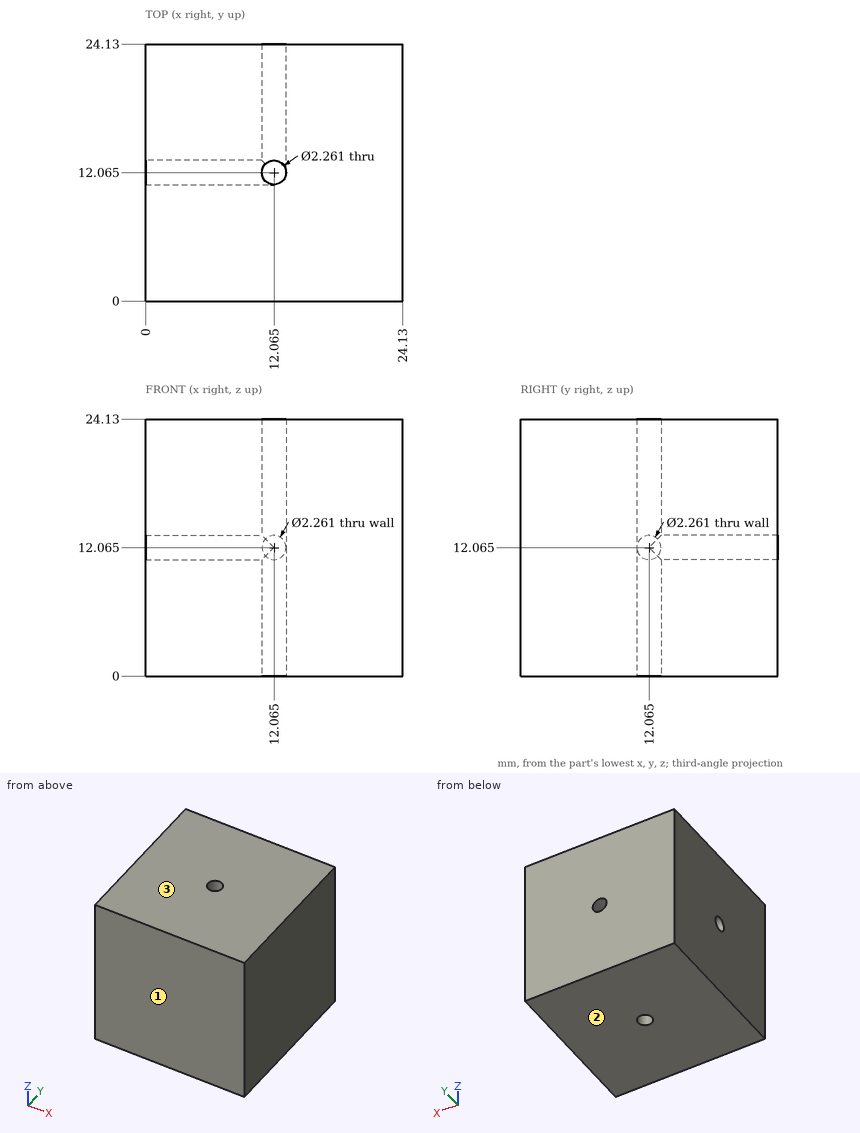
Input: dimensioned drawing with shaded views. Units: mm. Origin: part minimum x, y, z. Coordinates: 2 decimals unless noted, no trailing zeros. Return JSON: item names as keys, results as strings. Group by question number.
1. Material intervals for line 1 along Y through (x, z) = (13, 2.5); line 2 along Z through (x, y) = (11.5, 23) (1 decimal); line 3 along Z through (x, y) = (12.25, 17.5), sorted ascending. Write a range as [from, to].
2. Pin query (flat end, axial travel): pin 1 (2 mm diameter, centred on x = 12.065, y = 12.065, fed in from -Z). Return the tip coordinate at first contact, or that it passes through.
3. Pull-direction query (Z, two-part tool) for the marked faces 1, 2 and 3; classes: pulls with the +Z half, pulls with the -Z half, needs draft (parallel to the pull), parting line crosses it, or undercut.
Resolved:
{
 "1": {"line 1": "y = [0, 11.43], [12.7, 24.13]", "line 2": "z = [0, 11.1], [13, 24.1]", "line 3": "z = [0, 10.95], [13.18, 24.13]"},
 "2": {"pin 1": "passes through"},
 "3": {"face 1": "needs draft", "face 2": "pulls with the -Z half", "face 3": "pulls with the +Z half"}
}
